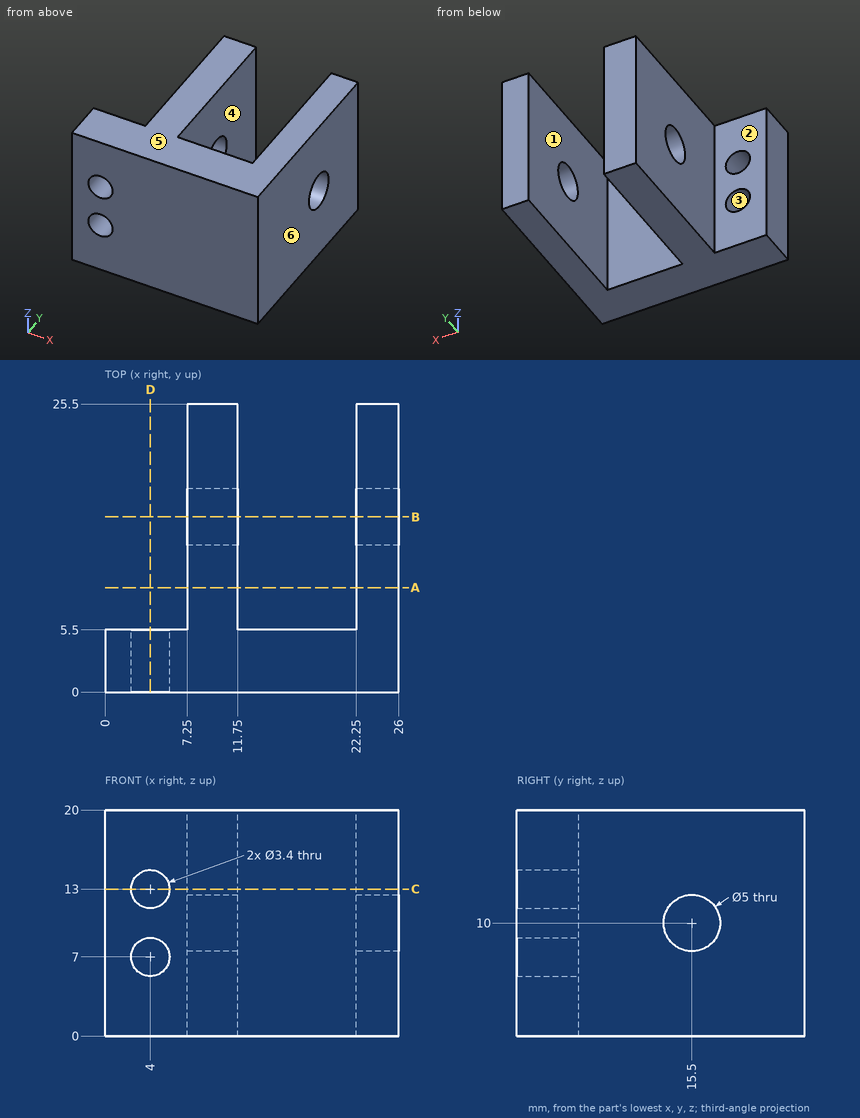
Study the drawing (mm; zero at the part's minimum x, y, z) and answer. A direction names the side the tool comes from. Round coordinates to 2 decimals unless told otherwise and drop trailing zeros. Write each loop counter-clockwise with the first axis right and the second up, starting at its lowest first coordinate (ties: lowest second). Pieces come first, ordered by that corner, then holes. Notation, with made-up numbers: (41, 45) -> (52, 45) arc R19 ccw to (52, 67) -> close; hole circle Ø11 at (64, 17). An arc over 180 degrees is marked (long way). Use CSV: the item, a comma, the result in double quotes. Start each with the question number.
(1) Each of these flat-tipped pins is pushed along its axis until it touches: pin 1 (5.5 mm diameter, centred on x = 4, z = 13, fed in from +Y); pin 2 (3 mm diameter, centred on x = 4, z = 7, fed in from +Y); pin 3 (8 mm diameter, centred on y = 15.5, z = 10, fed in from -X). Where does it stop, or does it pass through?
(2) The mould has two halves that part along X. Classify the marked faces 4, 5 and 6: released by +X, released by -X, zero draft, split by the parting line, or undercut.
(3) Section D-D on x = 4 is taken. Give the vertices of the cut face in (y, z).
(4) Section A-A on y = 9.25 is taken. Give the vertices of the cut face in (x, z), then the cut area to 3 significant figures.
(5) Section C-C on z = 13 is taken. Give the vertices of the cut face in (x, y), then the cut area to 3 significant figures.
(6) Consider L1, parallel to X at y = 10.5, z = 2.75; L2, parallel to Y at x = 9.05, z = 10; L3, parallel to X at y = 1.55, z = 7. Determine where each line is inside the solid, lowest interval first. Write a range as from..to.
(7) Which of the six approach directions +Z, -Z, +X, -X, +Y, -Y give full straight-line access (tool end or side, diameter ignored) to the marked faces 1, 2 and 3?
(8) Section B-B on y = 15.5 is taken. Give the vertices of the cut face in (x, z), then the cut area to 3 significant figures.
A:
1,pin 1,"stops at y = 5.5"
1,pin 2,"passes through"
1,pin 3,"stops at x = 7.25"
2,face 4,"undercut"
2,face 5,"zero draft"
2,face 6,"released by +X"
3,outline,"(0, 0) -> (5.5, 0) -> (5.5, 5.3) -> (0, 5.3) -> close; (0, 8.7) -> (5.5, 8.7) -> (5.5, 11.3) -> (0, 11.3) -> close; (0, 14.7) -> (5.5, 14.7) -> (5.5, 20) -> (0, 20) -> close"
4,outline,"(7.25, 0) -> (11.75, 0) -> (11.75, 20) -> (7.25, 20) -> close; (22.25, 0) -> (26, 0) -> (26, 20) -> (22.25, 20) -> close"
4,area,"165 mm²"
5,outline,"(0, 0) -> (2.3, 0) -> (2.3, 5.5) -> (0, 5.5) -> close; (5.7, 0) -> (26, 0) -> (26, 25.5) -> (22.25, 25.5) -> (22.25, 5.5) -> (11.75, 5.5) -> (11.75, 25.5) -> (7.25, 25.5) -> (7.25, 5.5) -> (5.7, 5.5) -> close"
5,area,"289 mm²"
6,L1,"x = 7.25..11.75, 22.25..26"
6,L2,"y = 0..13, 18..25.5"
6,L3,"x = 0..2.3, 5.7..26"
7,face 1,"+Z, -Z, +Y"
7,face 2,"+Z, -Z, -X, +Y"
7,face 3,"+Y, -Y"
8,outline,"(7.25, 0) -> (11.75, 0) -> (11.75, 7.5) -> (7.25, 7.5) -> close; (7.25, 12.5) -> (11.75, 12.5) -> (11.75, 20) -> (7.25, 20) -> close; (22.25, 0) -> (26, 0) -> (26, 7.5) -> (22.25, 7.5) -> close; (22.25, 12.5) -> (26, 12.5) -> (26, 20) -> (22.25, 20) -> close"
8,area,"124 mm²"
